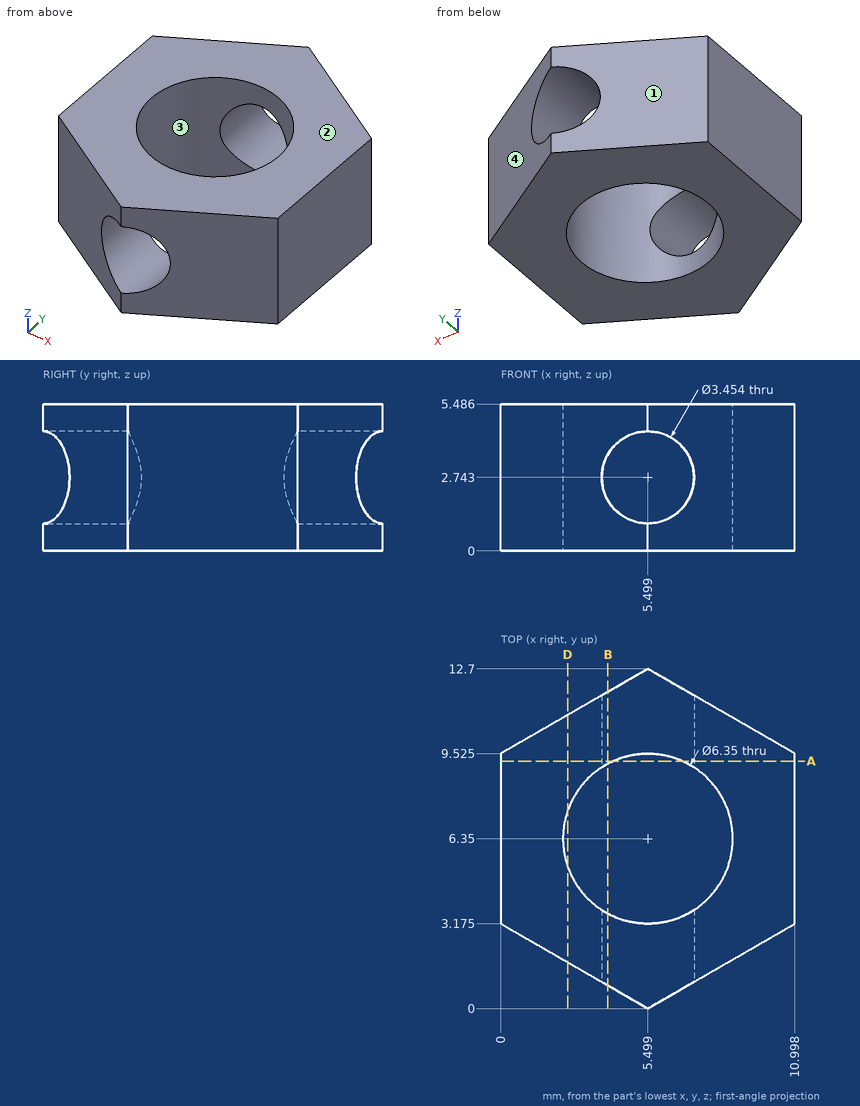
Check sheet for the drawn part. Datum: minimum x, y, z corner. Units: mm. Round coordinates to 2 decimals unless told otherwise and drop trailing zeros. Write each loop counter-clockwise with the first axis right and the second up, starting at its lowest first coordinate (ties: lowest second). Pieces come first, ordered by that corner, then holes. Notation, with made-up numbers: (25, 81) - (84, 81) arc R8 cw to (84, 94) - close; hole circle Ø3 at (23.25, 45.25). An arc over 180 degrees is marked (long way). Write each question's results on one line, items separated by ' | '.
(1) Sectioned sample at B-B, the plane x = 4. Enter the section's corners in (y, z) (1 decimal).
Computed:
outline: (0.9, 0) - (3.6, 0) - (3.6, 1.9) - (0.9, 1.9) - close; (0.9, 3.6) - (3.6, 3.6) - (3.6, 5.5) - (0.9, 5.5) - close; (9.1, 0) - (11.8, 0) - (11.8, 1.9) - (9.1, 1.9) - close; (9.1, 3.6) - (11.8, 3.6) - (11.8, 5.5) - (9.1, 5.5) - close
(2) Thickness scan on probe 1 along Z at (x, y) = (5.5, 2.25); probe 2 along X at (y, z) = (11.25, 2.5) (1 decimal); probe 3 along Y at (x, z) = (2.75, 3.55) (1 decimal). Record the ranges inside material, lowest first. Write a range as from..to.
Computed:
probe 1: z = 0..1.02, 4.47..5.49 | probe 2: x = 3..3.8, 7.2..8 | probe 3: y = 1.6..4.8, 7.9..11.1
(3) Sectioned sample at D-D, the plane x = 2.5. Enter the section's corners in (y, z).
Computed:
outline: (1.73, 0) - (5.31, 0) - (5.31, 5.49) - (1.73, 5.49) - close; (7.39, 0) - (10.97, 0) - (10.97, 5.49) - (7.39, 5.49) - close
(4) Draft check along X on the marked faces 1, 2, 3 and 4. Enter one of: pulls with the +X half, pulls with the -X half, needs draft (parallel to the pull), parting line crosses it, or undercut.
Computed:
face 1: pulls with the -X half | face 2: needs draft | face 3: undercut | face 4: pulls with the +X half
(5) Sectioned sample at A-A, the plane y = 9.25. Enter the section's corners in (x, z) (1 decimal), plus the area to 3 significant figures.
Computed:
outline: (0, 0) - (4.2, 0) - (4.2, 1.6) arc R1.7 cw to (4.2, 3.9) - (4.2, 5.5) - (0, 5.5) - close; (6.8, 0) - (11, 0) - (11, 5.5) - (6.8, 5.5) - (6.8, 3.9) arc R1.7 cw to (6.8, 1.6) - close | area: 44.8 mm^2
(6) Depth check by flat-ended pin: pin 1 Ø5 at (x, y) = (5.5, 6.35) entering from -Z; pin 2 Ø1 at (x, z) = (1.5, 1) entering from -Y; pin 3 Ø3 at (x, z) = (3.5, 2.5) entering from +Y (1 decimal); pin 4 Ø2 at (y, z) = (11, 2.5) entering from -X (1 decimal). Enter the tip coordinate at first touch or a pass-through.
Computed:
pin 1: passes through | pin 2: stops at y = 2.02 | pin 3: stops at y = 12.1 | pin 4: stops at x = 0.8
